Verification items for the finished model (mm, model axes). Face numbers are marked on the shaded views. A direction names the side the tool comes from. Coordinates: 2 decimals unless noted, no trailing zeros. Loops run counter-clockwise (first coordinate to the right, second up) from the corner with the lowest first, then second, coordinate; pieces in that order, holes last. Notation, with made-up numbers: (84, -4.75) - (110, -4.75) arc R19 ccw to (110, 2.25) - close; hole circle Ø7 at (-31.75, 48). An arc over 180 degrees is marked (long way). One line per item, written item: value. Start each with the question number.
(1) Section check D-D (z = -22). Record the boundary of the cut face in (x, y), plus the area to 3 significant figures.
(2) Section check B-B (z = 0). Record the boundary of the cut face in (x, y).
(3) Section check A-A (y = 0). Record the boundary of the cut face in (x, z).
(4) Gauge pin test, flat ends, axial feed: P1, Ø5, axis at y = -12.37, z = -12.37, coming from the +X side; P2, Ø3.5, axis at x = 60, z = 27, coming from the -Y side. Record the tip position at first contact, or that the pin passes through.
(5) Set-up check for the marked faces 4, 5 and 6: record each of +Z, -Z, +X, -X, +Y, -Y from which the full face is reachable in a straight line by a thin tool's end or side.
(6) Thickness scan on probe 1 along Y at (x, z) = (11, -32); probe 2 along Z at (x, y) = (20, -10.5); probe 3 along Z at (x, y) = (7, -24.5). Record the ranges inside material, lowest first. Write a range as [from, to].
(7) Draft check along Y on the marked faces 1, 2 and 3. Enter one of: +Y half, -Y half, draft (parallel to the pull), parting line (faces both ways), or undercut.
(8) Section check C-C (x = 15). Count the separate pieces of the cut face and the enclosed holes in it, plus the area to 3 significant figures.
```python
from build123d import *

# Parameters (mm, degrees)
SKETCH1_W           = 75
SKETCH1_H           = 60
BOSS_EXTRUDE1_DEPTH = 75
SKETCH2_R           = 23.1
CUT_EXTRUDE1_DEPTH  = 70
SKETCH3_R           = 2.25
CUT_EXTRUDE2_DEPTH  = 90.057565653
CUT_EXTRUDE3_REACH  = 105.108
SKETCH4_R           = 2.25


with BuildPart() as part:
    # Sketch1 → Boss-Extrude1 (new body)
    with BuildSketch(Plane(origin=(0, 0, 0), x_dir=(0, 0, -1), z_dir=(1, 0, 0))):
        Rectangle(SKETCH1_W, SKETCH1_H)
    extrude(amount=BOSS_EXTRUDE1_DEPTH)

    # Sketch2 → Cut-Extrude1 (cut)
    with BuildSketch(Plane(origin=(75, 0, 0), x_dir=(0, 0, -1), z_dir=(1, 0, 0))):
        Circle(SKETCH2_R)
    extrude(amount=-CUT_EXTRUDE1_DEPTH, mode=Mode.SUBTRACT)

    # Sketch3 → Cut-Extrude2 (cut, through all)
    with BuildSketch(Plane.ZY):
        with Locations((-12.374368671, 12.374368671)):
            Circle(SKETCH3_R)
        with Locations((12.374368671, 12.374368671)):
            Circle(SKETCH3_R)
        with Locations((12.374368671, -12.374368671)):
            Circle(SKETCH3_R)
        with Locations((-12.374368671, -12.374368671)):
            Circle(SKETCH3_R)
        with BuildLine():
            Line((-5.07937004, 12.4), (5.07937004, 12.4))
            ThreePointArc((5.07937004, 12.4), (13.4, 0), (5.07937004, -12.4))
            Line((5.07937004, -12.4), (-5.07937004, -12.4))
            ThreePointArc((-5.07937004, -12.4), (-13.4, 0), (-5.07937004, 12.4))
        make_face()
        with BuildLine():
            Line((32.5, -25), (14.5, -25))
            Line((14.5, -25), (14.5, -24.069898213))
            ThreePointArc((14.5, -24.069898213), (23.416139376, -15.533654327), (27.813845473, -4))
            Line((27.813845473, -4), (32.5, -4))
            Line((32.5, -4), (32.5, -25))
        make_face()
        with BuildLine():
            Line((32.5, 25), (14.5, 25))
            Line((14.5, 25), (14.5, 24.069898213))
            ThreePointArc((14.5, 24.069898213), (23.416139376, 15.533654327), (27.813845473, 4))
            Line((27.813845473, 4), (32.5, 4))
            Line((32.5, 4), (32.5, 25))
        make_face()
        with BuildLine():
            Line((-32.5, -25), (-32.5, -4))
            Line((-32.5, -4), (-27.813845473, -4))
            ThreePointArc((-27.813845473, -4), (-23.416139376, -15.533654327), (-14.5, -24.069898213))
            Line((-14.5, -24.069898213), (-14.5, -25))
            Line((-14.5, -25), (-32.5, -25))
        make_face()
        with BuildLine():
            Line((-32.5, 4), (-27.813845473, 4))
            ThreePointArc((-27.813845473, 4), (-23.416139376, 15.533654327), (-14.5, 24.069898213))
            Line((-14.5, 24.069898213), (-14.5, 25))
            Line((-14.5, 25), (-32.5, 25))
            Line((-32.5, 25), (-32.5, 4))
        make_face()
    extrude(amount=-CUT_EXTRUDE2_DEPTH, mode=Mode.SUBTRACT)

    # Sketch4 → Cut-Extrude3 (cut, up to next)
    with BuildSketch(Plane.XZ.offset(30), mode=Mode.PRIVATE) as cut_extrude3_sk1:
        with Locations(Location((60, 27, 0), (0, 0, 270))):
            Circle(SKETCH4_R)
    cut_extrude3_tool1 = extrude(cut_extrude3_sk1.sketch, amount=-CUT_EXTRUDE3_REACH, mode=Mode.PRIVATE) & part.part
    # Sketch4 → Cut-Extrude3 (cut, up to next)
    with BuildSketch(Plane.XZ.offset(30), mode=Mode.PRIVATE) as cut_extrude3_sk2:
        with Locations(Location((15, 27, 0), (0, 0, 270))):
            Circle(SKETCH4_R)
    cut_extrude3_tool2 = extrude(cut_extrude3_sk2.sketch, amount=-CUT_EXTRUDE3_REACH, mode=Mode.PRIVATE) & part.part
    # Sketch4 → Cut-Extrude3 (cut, up to next)
    with BuildSketch(Plane.XZ.offset(30), mode=Mode.PRIVATE) as cut_extrude3_sk3:
        with Locations(Location((60, -27, 0), (0, 0, 270))):
            Circle(SKETCH4_R)
    cut_extrude3_tool3 = extrude(cut_extrude3_sk3.sketch, amount=-CUT_EXTRUDE3_REACH, mode=Mode.PRIVATE) & part.part
    # Sketch4 → Cut-Extrude3 (cut, up to next)
    with BuildSketch(Plane.XZ.offset(30), mode=Mode.PRIVATE) as cut_extrude3_sk4:
        with Locations(Location((15, -27, 0), (0, 0, 270))):
            Circle(SKETCH4_R)
    cut_extrude3_tool4 = extrude(cut_extrude3_sk4.sketch, amount=-CUT_EXTRUDE3_REACH, mode=Mode.PRIVATE) & part.part
    add(cut_extrude3_tool1.solids().sort_by_distance((60, -30, 27))[0], mode=Mode.SUBTRACT)
    add(cut_extrude3_tool2.solids().sort_by_distance((15, -30, 27))[0], mode=Mode.SUBTRACT)
    add(cut_extrude3_tool3.solids().sort_by_distance((60, -30, -27))[0], mode=Mode.SUBTRACT)
    add(cut_extrude3_tool4.solids().sort_by_distance((15, -30, -27))[0], mode=Mode.SUBTRACT)


solid = part.part
```
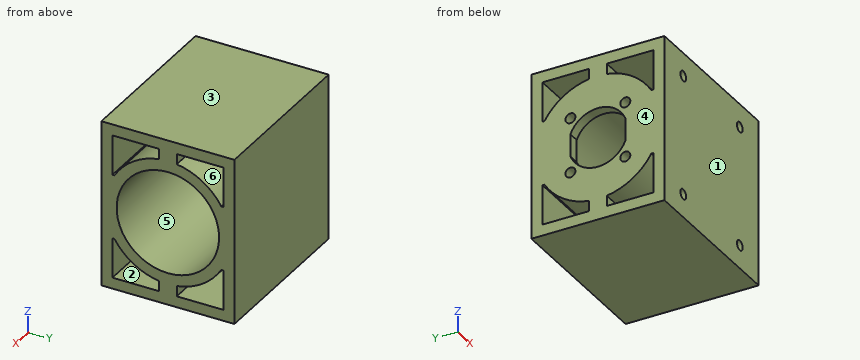
Responses:
1. outline: (0, -30) - (75, -30) - (75, -25) - (0, -25) - close; (0, -17.48) - (75, -17.48) - (75, -7.04) - (5, -7.04) - (5, 7.04) - (75, 7.04) - (75, 17.48) - (0, 17.48) - close; (0, 25) - (75, 25) - (75, 30) - (0, 30) - close
1. area: 2,390 mm²
2. outline: (0, -30) - (75, -30) - (75, -23.1) - (5, -23.1) - (5, -12.4) - (0, -12.4) - close; (0, 12.4) - (5, 12.4) - (5, 23.1) - (75, 23.1) - (75, 30) - (0, 30) - close
3. outline: (0, -37.5) - (75, -37.5) - (75, -23.1) - (5, -23.1) - (5, -13.4) - (0, -13.4) - close; (0, 13.4) - (5, 13.4) - (5, 23.1) - (75, 23.1) - (75, 37.5) - (0, 37.5) - close
4. P1: stops at x = 5
4. P2: stops at y = -12.33
5. face 4: +Z, -Z, -X, +Y, -Y
5. face 5: +X
5. face 6: +X, -X
6. probe 1: y = [-30, -25], [-4, 4], [25, 30]
6. probe 2: z = [-37.5, -32.5], [-26.06, -20.58], [20.58, 26.06], [32.5, 37.5]
6. probe 3: z = [-37.5, -32.5], [-14.5, 14.5], [32.5, 37.5]
7. face 1: -Y half
7. face 2: undercut
7. face 3: draft
8. separate pieces: 1
8. enclosed holes: 3
8. area: 1,980 mm²
